Geometry check sheet. Reference: the model listing, model coordinates, mm. A direction names the side the tool comes from. Round coordinates to 2 decimals unless told otherwise and drop trailing zeros. Loops run counter-clockwise (first coordinate to the right, second up) from the corner with the lowest first, then second, coordinate; pieces in that order, holes last. Notation, with made-up numbers: (88, -36) - (139, -36) arc R27 ccw to (139, -14) - close; hole circle Ø9 at (57.5, 2). An arc over 180 degrees is marked (long way). Answer as CSV lines item,"result". Start each with the question number.
1) Cross-section at D-D on z = -48.5. Record the boundary of the cut face in (x, y).
2) Cross-section at A-A on z = 6. Record the boundary of the cut face in (x, y), and give its area (3 significant figures).
3) Cross-section at B-B on x = 6. Record the boundary of the cut face in (y, z).
4) Thickness scan on line 1 along X through (y, z) = (-1.4, 0); line 2 along X through (y, z) = (-2.65, -0.5). Record the ranges inside material, lowest first.
5) Access from +Z, -Z, +X, -X, +Y, -Y to the whole of each face (thin tool, end or side, straight path). Record for faces 5 (the flat face through (-10, -1, -12.5)), 6 (the flat face through (0, -2, -23)), 7 (the cylindrical face through (-21.99, -1.01, 9.65)), 8 (the flat face through (-12.95, -1, 10)), 9 (the flat face through (-8, -2, 9)).
6) Cross-section at C-C on y = -1.05. Record the boundary of the cut face in (x, z), and give its area (3 significant figures).
7) Draft check along X on faces 1 (the flat face through (-2.95, -3, -23)), 2 (the flat face through (-20, -2, -5)), 3 (the flat face through (12.95, -1, 10)), 4 (the cylindrical face through (-22.15, -1.01, -9.49)). Enter one of: released by +X, released by -X, zero draft, split by the parting line, or undercut.
8) Depth check by flat-ended pin: P1, Ø1.6, axis at y = -0.5, z = 11, coming from the -X side; P2, Ø1.7, axis at x = -0.5, z = -27.5, coming from the -Y side; P3, Ø2, axis at y = -3.5, z = -34, coming from the +X side. Enter the tip coordinate at first touch or a pass-through.
from build123d import *

# Parameters (mm, degrees)
F0_W     = 5.54
F0_H     = 25
F1_DEPTH = 2
F2_R     = 10
F3_DEPTH = 5
F5_DEPTH = 47.79
F6_R     = 1


# Not quite as in the source:
# - a feature of the source that left no trace in its solid (it failed there, or was rolled back) is left out


with BuildPart() as f1:
    # F0 (on Front) → F1 (new body)
    with BuildSketch(Plane.XZ):
        with BuildLine():
            Line((4.49, -12.5), (25, -12.5))
            Line((25, -12.5), (25, 12.5))
            Line((25, 12.5), (13.95, 12.5))
            Line((13.95, 12.5), (13.95, 8.0380345856))
            ThreePointArc((13.95, 8.0380345856), (19.0208319035, 5.3623688795), (21.05, 0))
            ThreePointArc((21.05, 0), (7.2224350724, -5.7275649276), (12.95, 8.1))
            Line((12.95, 8.1), (12.95, 12.5))
            Line((12.95, 12.5), (4.49, 12.5))
            Line((4.49, 12.5), (4.49, 0))
            Line((4.49, 0), (4.49, -12.5))
        make_face()
        with BuildLine():
            ThreePointArc((-12.95, 8.1), (-7.2224350724, 5.7275649276), (-4.85, 0))
            Line((-4.85, 0), (-4.85, 12.5))
            Line((-4.85, 12.5), (-12.95, 12.5))
            Line((-12.95, 12.5), (-12.95, 8.1))
        make_face()
        with BuildLine():
            Line((-25, -12.5), (-4.85, -12.5))
            Line((-4.85, -12.5), (-4.85, 0))
            ThreePointArc((-4.85, 0), (-18.3123688795, -6.0708319035), (-13.95, 8.0380345856))
            Line((-13.95, 8.0380345856), (-13.95, 12.5))
            Line((-13.95, 12.5), (-25, 12.5))
            Line((-25, 12.5), (-25, -12.5))
        make_face()
        Polygon((-4.85, -12.5), (-2.95, -12.5), (-2.95, 12.5), (-4.85, 12.5), (-4.85, 0), align=None)
        with Locations((-0.18, 0)):
            Rectangle(F0_W, F0_H)
        Polygon((2.59, -12.5), (4.49, -12.5), (4.49, 0), (4.49, 12.5), (2.59, 12.5), align=None)
    extrude(amount=F1_DEPTH)

    # F2
    f2_edges = [f1.edges().sort_by_distance(p)[0] for p in [
        (25, -1, -12.5),
        (25, -1, 12.5),
        (-25, -1, 12.5),
        (-25, -1, -12.5),
    ]]
    fillet(f2_edges, radius=F2_R)

    # F0 (on Front) → F3 (join)
    with BuildSketch(Plane.XZ):
        Polygon((2.59, -12.5), (4.49, -12.5), (4.49, 0), (4.49, 12.5), (2.59, 12.5), align=None)
        Polygon((-4.85, -12.5), (-2.95, -12.5), (-2.95, 12.5), (-4.85, 12.5), (-4.85, 0), align=None)
    extrude(amount=F3_DEPTH)

    # F4 (on face) → F5 (join)
    with BuildSketch(Plane(origin=(0, 0, -12.5), x_dir=(1, 0, 0), z_dir=(0, 0, -1))):
        Polygon((-2.95, 5), (-4.85, 5), (-4.85, 0), (4.49, 0), (4.49, 2), (4.49, 5), (2.59, 5), (2.59, 2), (-2.95, 2), align=None)
    extrude(amount=F5_DEPTH)

    # F6
    f6_edges = [f1.edges().sort_by_distance(p)[0] for p in [
        (-3.9, -5, 12.5),
        (3.54, -5, 12.5),
    ]]
    fillet(f6_edges, radius=F6_R)


solid = f1.part
Answer block:
1,outline,"(-4.85, -5) - (-2.95, -5) - (-2.95, -2) - (2.59, -2) - (2.59, -5) - (4.49, -5) - (4.49, 0) - (-4.85, 0) - close"
2,outline,"(-24.37, -2) - (-18.39, -2) - (-18.39, 0) - (-24.37, 0) - close; (-7.51, -2) - (-4.85, -2) - (-4.85, -5) - (-2.95, -5) - (-2.95, -2) - (2.59, -2) - (2.59, -5) - (4.49, -5) - (4.49, -2) - (7.51, -2) - (7.51, 0) - (-7.51, 0) - close; (18.39, -2) - (24.37, -2) - (24.37, 0) - (18.39, 0) - close"
2,area,"65.3 mm^2"
3,outline,"(-2, -12.5) - (0, -12.5) - (0, -4.16) - (-2, -4.16) - close; (-2, 4.16) - (0, 4.16) - (0, 12.5) - (-2, 12.5) - close"
4,line 1,"x = -25 to -21.05, -4.85 to 4.85, 21.05 to 25"
4,line 2,"x = -4.85 to -2.95, 2.59 to 4.49"
5,face 5,"-Z, -X, +Y, -Y"
5,face 6,"+Z, -Z, -Y"
5,face 7,"+Z, -X, +Y, -Y"
5,face 8,"+Z, +Y, -Y"
5,face 9,"+Z, -Z, -X, -Y"
6,outline,"(-25, -2.5) arc R10 ccw to (-15, -12.5) - (-4.85, -12.5) - (-4.85, -60.29) - (4.49, -60.29) - (4.49, -12.5) - (15, -12.5) arc R10 ccw to (25, -2.5) - (25, 2.5) arc R10 ccw to (15, 12.5) - (13.95, 12.5) - (13.95, 8.04) arc R8.1 cw (long way) to (12.95, 8.1) - (12.95, 12.5) - (-12.95, 12.5) - (-12.95, 8.1) arc R8.1 cw (long way) to (-13.95, 8.04) - (-13.95, 12.5) - (-15, 12.5) arc R10 ccw to (-25, 2.5) - close"
6,area,"1,190 mm^2"
7,face 1,"undercut"
7,face 2,"zero draft"
7,face 3,"undercut"
7,face 4,"released by -X"
8,P1,"stops at x = -21.38"
8,P2,"stops at y = -2"
8,P3,"stops at x = 4.49"
